Check sheet for the drawn part. Datum: minimum x, y, z corner. Units: mm. A direction names the side the tool comes from. Round coordinates to 2 decimals unless told otherwise and drop trailing zeros. Write each loop counter-clockwise with the first axis right and the second up, starting at its lowest first coordinate (ties: lowest second). Pieces come first, ordered by that corner, then holes. Notation, with made-up numbers: (50, -34.5) - (95, -34.5) arc R11 ccw to (95, -13.5) - close; hole circle Ø1 at (75, 26.5). An arc over 180 degrees is marked (long way). Answer as a JSON object with one key per item and string values.
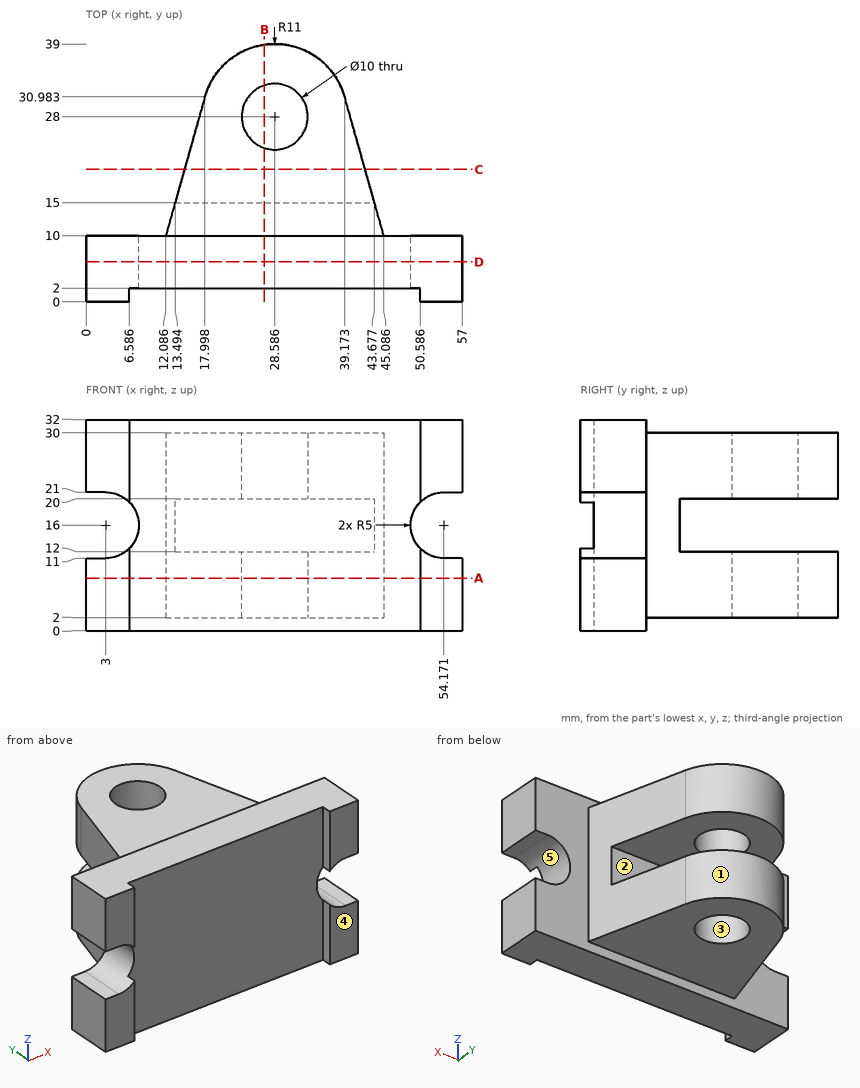
1. Material ranges on probe 1 along Z at (x, y) = (19, 29); probe 2 along Z at (x, y) = (3, 3.5); probe 3 along Y at (x, z) = (6, 7), recorded low to high. Write a range as from..to.
Completed:
{"probe 1": "z = 2..12, 20..30", "probe 2": "z = 0..11, 21..32", "probe 3": "y = 0..10"}
2. Mould release check, pull along X, two halves, no side actions. Record for the marked faces 3, 4 and 5: released by +X, released by -X, zero draft, split by the parting line, or undercut.
Completed:
{"face 3": "undercut", "face 4": "zero draft", "face 5": "released by +X"}
3. Cross-section at D-D (y = 6). Record the boundary of the cut face in (x, z).
Completed:
{"outline": "(0, 0) - (57, 0) - (57, 11) - (54.17, 11) arc R5 cw to (54.17, 21) - (57, 21) - (57, 32) - (0, 32) - (0, 21) - (3, 21) arc R5 cw to (3, 11) - (0, 11) - close"}
4. Go/stop test with flat-tipped pins: pin 1 (3 mm diameter, centred on x = 37.5, z = 6.5, fed in from -Y); pin 2 (11.5 mm diameter, centred on x = 28.59, y = 28, fed in from +Z); pin 3 (8 mm diameter, centred on y = 25.5, z = 8.5, fed in from -X). Record where each tip stops, or that it passes through.
Completed:
{"pin 1": "stops at y = 2", "pin 2": "stops at z = 30", "pin 3": "stops at x = 15.33"}
5. Cross-section at A-A (z = 8). Record the boundary of the cut face in (x, y) (1 decimal).
Completed:
{"outline": "(0, 0) - (6.6, 0) - (6.6, 2) - (50.6, 2) - (50.6, 0) - (57, 0) - (57, 10) - (45.1, 10) - (39.2, 31) arc R11 ccw to (18, 31) - (12.1, 10) - (0, 10) - close; hole circle Ø10 at (28.6, 28)"}
6. Access from +Z, -Z, +X, -X, +Y, -Y to the whole of each face (thin tool, end or side, straight path). Record for the marked faces 1 and 2.
Completed:
{"face 1": "+Z, -Z, +Y", "face 2": "+X, -X, +Y"}
7. Cross-section at B-B (x = 27). Record the boundary of the cut face in (y, z) (1 decimal).
Completed:
{"outline": "(2, 0) - (10, 0) - (10, 2) - (23.3, 2) - (23.3, 12) - (15, 12) - (15, 20) - (23.3, 20) - (23.3, 30) - (10, 30) - (10, 32) - (2, 32) - close; (32.7, 2) - (38.9, 2) - (38.9, 12) - (32.7, 12) - close; (32.7, 20) - (38.9, 20) - (38.9, 30) - (32.7, 30) - close"}
8. Cross-section at C-C (y = 20). Record the boundary of the cut face in (x, z).
Completed:
{"outline": "(14.9, 2) - (42.27, 2) - (42.27, 12) - (14.9, 12) - close; (14.9, 20) - (42.27, 20) - (42.27, 30) - (14.9, 30) - close"}
